Model file for the job. Use its own axes, mm. Face numbers are marked on the shaded views. A direction names the side the tool comes from. Round coordinates to 2 decimals unless told otherwise and drop trailing zeros. Order: outer loops, then holes, each group sorted by start corner. A loop starts at its lowest first (then second) coordinate and runs counter-clockwise, first axis right, second up. Notation, with made-up numbers: M -32.5,-37.75 L 10.5,-37.75 A8 ccw 10.5,-28.75 Z; hole C 39,74.25 d10. An arc over 180 degrees is marked long. Return JSON: item names as keys, results as strings. Group by question number.
Item 1: Slice it at D-D on y = 27.5. Write the cut outline in (x, z), then the cut area to 3 significant figures.
Item 2: Pull direction Z, two halves, no side cores. Call the marked faces 1, 2 and 3: pulls with the +Z half, pulls with the -Z half, needs draft (parallel to the pull), parting line crosses it, or undercut.
Item 3: Slice it at C-C on x = 7.5. Write the cut outline in (y, z).
Item 4: Slice it at A-A on x = -31.5. Write the cut outline in (y, z), then the cut area to 4 significant figures.
Item 5: Slice it at B-B on z = -40.5. Write the cut outline in (x, y), then the cut area to 3 significant figures.
Item 6: Probe line 1 along Z through (x, y) = (-55.5, 3.85); line 2 along X through (y, z) = (3.85, 69.5); line 3 along Y through (x, z) = (-22.5, 65.5). List the from-to ranges inside material, lowest first.
Item 7: Pin check, flat tips, straight feed: pin 1 Ø4.5 at (x, z) = (-55.5, 5.5) entering from -Y; pin 2 Ø13 at (y, z) = (38, 31.5) entering from -X; pin 3 Ø2 at (x, z) = (-38.5, 9.5) entering from +Y. Stop position of each tip, or through.
Item 8: Which spindle directions (+Z, -Z, +X, -X, +Y, -Y) get a long thin tool onto all of the face, cutting with end or side? Do the marked faces 4, 5 and 6. Say none if no direction does.
from build123d import *

# Parameters (mm, degrees)
SKETCH1_W                                           = 52
SKETCH1_H                                           = 100
BOSS_EXTRUDE1_DEPTH                                 = 5
BOSS_EXTRUDE3_DEPTH                                 = 2.5
SKETCH7_R                                           = 2.25
BOSS_EXTRUDE4_DEPTH                                 = 2.5
FILLET2_R                                           = 0.25
SKETCH9_W                                           = 52
SKETCH9_H                                           = 4
BOSS_EXTRUDE5_DEPTH                                 = 50
BOSS_EXTRUDE7_DEPTH                                 = 52
CUT_EXTRUDE3_DEPTH                                  = 52
CUT_EXTRUDE4_DEPTH                                  = 2.5
BOSS_EXTRUDE8_DEPTH                                 = 52
BOSS_EXTRUDE9_DEPTH                                 = 4
LPATTERN1_COUNT                                     = 2
LPATTERN1_PITCH                                     = 48
SKETCH18_R                                          = 11.5
CUT_EXTRUDE5_DEPTH                                  = 4
CSK_FOR_M3_COUNTERSUNK_FLAT_HEAD_SCREW1_D           = 3.4
CSK_FOR_M3_COUNTERSUNK_FLAT_HEAD_SCREW1_DEPTH       = 5
CSK_FOR_M3_COUNTERSUNK_FLAT_HEAD_SCREW1_CSINK_D     = 6.3
CSK_FOR_M3_COUNTERSUNK_FLAT_HEAD_SCREW1_CSINK_ANGLE = 90
CSK_FOR_M3_COUNTERSUNK_FLAT_HEAD_SCREW1_TIP         = 1.021463052
BOSS_EXTRUDE10_DEPTH                                = 5
SKETCH23_R                                          = 1.75
CUT_EXTRUDE6_DEPTH                                  = 5
SKETCH24_W                                          = 6.6
SKETCH24_H                                          = 5.6
CUT_EXTRUDE7_DEPTH                                  = 2.5


with BuildPart() as part:
    # Sketch1 → Boss-Extrude1 (new body)
    with BuildSketch(Plane(origin=(0, 0, 0), x_dir=(1, 0, 0), z_dir=(0, 1, 0))):
        Rectangle(SKETCH1_W, SKETCH1_H)
    extrude(amount=BOSS_EXTRUDE1_DEPTH)

    # Sketch2 → Boss-Extrude3 (add)
    with BuildSketch(Plane(origin=(0, 5, 0), x_dir=(1, 0, 0), z_dir=(0, 1, 0))):
        with BuildLine():
            Line((-26, 50), (26, 50))
            Line((26, 50), (26, 30))
            ThreePointArc((26, 30), (0, 22.708313008), (-26, 30))
            Line((-26, 30), (-26, 50))
        make_face()
    extrude(amount=BOSS_EXTRUDE3_DEPTH)

    # Sketch7 → Boss-Extrude4 (add)
    with BuildSketch(Plane(origin=(0, 7.5, 0), x_dir=(1, 0, 0), z_dir=(0, 1, 0))):
        with Locations((-7.5, 40.5)):
            Circle(SKETCH7_R)
        with Locations((7.5, 40.5)):
            Circle(SKETCH7_R)
    extrude(amount=BOSS_EXTRUDE4_DEPTH)

    # Fillet2
    fillet2_edges = [part.edges().sort_by_distance(p)[0] for p in [
        (-9.75, 10, -40.5),
        (5.25, 10, -40.5),
    ]]
    fillet(fillet2_edges, radius=FILLET2_R)

    # Sketch9 → Boss-Extrude5 (add)
    with BuildSketch(Plane(origin=(0, 5, 0), x_dir=(1, 0, 0), z_dir=(0, 1, 0))):
        with Locations((0, -2)):
            Rectangle(SKETCH9_W, SKETCH9_H)
    extrude(amount=BOSS_EXTRUDE5_DEPTH)

    # Sketch10 → Boss-Extrude7 (add)
    with BuildSketch(Plane.ZY.offset(26)):
        Polygon((4, 25), (25.126220325, 64.732641679), (21.594429954, 66.61052793), (4, 33.520217873), align=None)
    extrude(amount=-BOSS_EXTRUDE7_DEPTH)

    # Sketch11 → Cut-Extrude3 (cut)
    with BuildSketch(Plane.ZY.offset(26)):
        Polygon((4, 33.520217873), (0, 25.498656006), (0, 55), (4, 55), align=None)
    extrude(amount=-CUT_EXTRUDE3_DEPTH, mode=Mode.SUBTRACT)

    # Sketch13 → Cut-Extrude4 (cut)
    with BuildSketch(Plane(origin=(0, 7.5, 0), x_dir=(1, 0, 0), z_dir=(0, 1, 0))):
        with BuildLine():
            Line((-14.75, 24.933450371), (-14.75, 50))
            Line((-14.75, 50), (-26, 50))
            Line((-26, 50), (-26, 30))
            ThreePointArc((-26, 30), (-20.531880242, 27.118381074), (-14.75, 24.933450371))
        make_face()
        with BuildLine():
            Line((26, 50), (14.75, 50))
            Line((14.75, 50), (14.75, 24.933450371))
            ThreePointArc((14.75, 24.933450371), (20.531880242, 27.118381074), (26, 30))
            Line((26, 30), (26, 50))
        make_face()
    extrude(amount=-CUT_EXTRUDE4_DEPTH, mode=Mode.SUBTRACT)

    # Sketch16 → Boss-Extrude8 (add)
    with BuildSketch(Plane.ZY.offset(26)):
        Polygon((4.234735781, 25.441473796), (42.679556541, 5), (37.679556541, 5), (4, 22.907737867), (4, 25), align=None)
    extrude(amount=-BOSS_EXTRUDE8_DEPTH)

    # Sketch17 → Boss-Extrude9 (add)
    with BuildSketch(Plane.ZY.offset(26)):
        Polygon((25.126220325, 64.732641679), (25.126220325, 5), (20.126220325, 5), (20.126220325, 55.329009352), align=None)
    boss_extrude9 = extrude(amount=-BOSS_EXTRUDE9_DEPTH)

    # LPattern1: Boss-Extrude9 ×2
    with Locations(*[(i * LPATTERN1_PITCH, 0, 0) for i in range(1, LPATTERN1_COUNT)]):
        add(boss_extrude9)

    # Sketch18 → Cut-Extrude5 (cut)
    with BuildSketch(Plane(origin=(0, 5.729899813, -10.776374221), x_dir=(-1, 0, 0), z_dir=(0, 0.469471563, -0.882947593))):
        with Locations((0, 45.951576073)):
            Circle(SKETCH18_R)
    extrude(amount=-CUT_EXTRUDE5_DEPTH, mode=Mode.SUBTRACT)

    # CSK for M3 Countersunk Flat Head Screw1
    with Locations(Plane(origin=(0, 5.729899813, -10.776374221), x_dir=(-1, 0, 0), z_dir=(0, 0.469471563, -0.882947593))):
        with Locations((-15.5, 61.451576073), (15.5, 61.451576073), (15.5, 30.451576073), (-15.5, 30.451576073)):
            CounterSinkHole(CSK_FOR_M3_COUNTERSUNK_FLAT_HEAD_SCREW1_D / 2, CSK_FOR_M3_COUNTERSUNK_FLAT_HEAD_SCREW1_CSINK_D / 2, depth=CSK_FOR_M3_COUNTERSUNK_FLAT_HEAD_SCREW1_DEPTH, counter_sink_angle=CSK_FOR_M3_COUNTERSUNK_FLAT_HEAD_SCREW1_CSINK_ANGLE)
            with Locations((0, 0, -(CSK_FOR_M3_COUNTERSUNK_FLAT_HEAD_SCREW1_DEPTH + CSK_FOR_M3_COUNTERSUNK_FLAT_HEAD_SCREW1_TIP / 2))):  # 118° drill point
                Cone(0, CSK_FOR_M3_COUNTERSUNK_FLAT_HEAD_SCREW1_D / 2, CSK_FOR_M3_COUNTERSUNK_FLAT_HEAD_SCREW1_TIP, mode=Mode.SUBTRACT)

    # Sketch22 → Boss-Extrude10 (add)
    with BuildSketch(Plane.XZ):
        Polygon((26, 75), (-61, 75), (-61, 0), (-26, 0), (-26, 50), (26, 50), align=None)
    extrude(amount=-BOSS_EXTRUDE10_DEPTH)

    # Sketch23 → Cut-Extrude6 (cut)
    with BuildSketch(Plane(origin=(0, 5, 0), x_dir=(1, 0, 0), z_dir=(0, 1, 0))):
        with Locations((-31.5, -5.5)):
            Circle(SKETCH23_R)
        with Locations((-55.5, -5.5)):
            Circle(SKETCH23_R)
        with Locations((-55.5, -69.5)):
            Circle(SKETCH23_R)
        with Locations((-31.5, -69.5)):
            Circle(SKETCH23_R)
    extrude(amount=-CUT_EXTRUDE6_DEPTH, mode=Mode.SUBTRACT)

    # Sketch24 → Cut-Extrude7 (cut)
    with BuildSketch(Plane.XZ):
        with Locations((-31.5, 69.5)):
            Rectangle(SKETCH24_W, SKETCH24_H)
        with Locations((-55.5, 69.5)):
            Rectangle(SKETCH24_W, SKETCH24_H)
        with Locations((-31.5, 5.5)):
            Rectangle(SKETCH24_W, SKETCH24_H)
        with Locations((-55.5, 5.5)):
            Rectangle(SKETCH24_W, SKETCH24_H)
    extrude(amount=-CUT_EXTRUDE7_DEPTH, mode=Mode.SUBTRACT)


solid = part.part
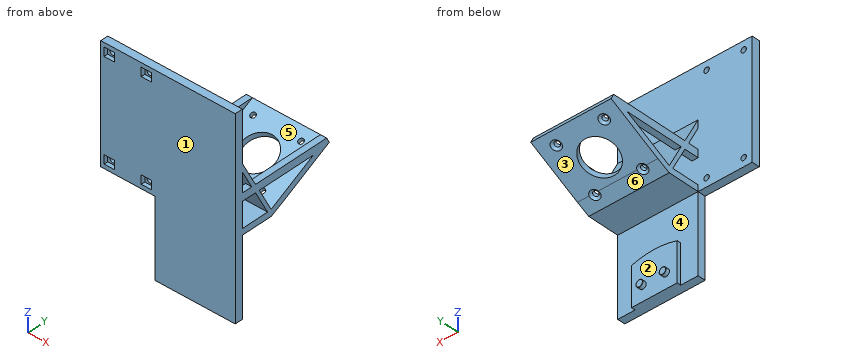
Output values:
{
 "1": {"outline": "M -26,1 L 26,1 L 26,5.33 L -26,5.33 Z; M -26,20.13 L -22,20.13 L -22,25.13 L -26,25.13 Z; M 22,20.13 L 26,20.13 L 26,25.13 L 22,25.13 Z", "area": "265 mm²"},
 "2": {"face 1": "needs draft", "face 2": "undercut", "face 3": "pulls with the -Z half"},
 "3": {"outline": "M 0,-50 L 7.5,-50 L 7.5,-42.75 L 9.75,-42.75 A0.25 ccw 10,-42.5 L 10,-38.5 A0.25 ccw 9.75,-38.25 L 7.5,-38.25 L 7.5,-23.27 L 5,-23.27 L 5,0 L 25.5,0 L 33.52,4 L 38.61,6.7 L 36.73,10.24 L 25.44,4.23 L 5,42.68 L 5,75 L 0,75 Z; M 52.12,18.42 L 54,14.89 L 66.61,21.59 L 64.73,25.13 Z; hole M 5,4 L 22.91,4 L 5,37.68 Z"},
 "4": {"outline": "M 0,0 L 5,0 L 5,3.75 L 2.5,3.75 L 2.5,2.7 L 0,2.7 Z; M 0,8.3 L 2.5,8.3 L 2.5,7.25 L 5,7.25 L 5,67.75 L 2.5,67.75 L 2.5,66.7 L 0,66.7 Z; M 0,72.3 L 2.5,72.3 L 2.5,71.25 L 5,71.25 L 5,75 L 0,75 Z", "area": "329.5 mm²"},
 "5": {"outline": "M -26,0 L 26,0 L 26,5 L 14.75,5 L 14.75,7.5 L 9.75,7.5 L 9.75,9.75 A0.25 ccw 9.5,10 L 5.5,10 A0.25 ccw 5.25,9.75 L 5.25,7.5 L -5.25,7.5 L -5.25,9.75 A0.25 ccw -5.5,10 L -9.5,10 A0.25 ccw -9.75,9.75 L -9.75,7.5 L -14.75,7.5 L -14.75,5 L -26,5 Z", "area": "356 mm²"},
 "6": {"line 1": "0 to 3.75, 7.25 to 67.75, 71.25 to 75", "line 2": "-61 to -57.25, -53.75 to -33.25, -29.75 to 26", "line 3": "0 to 5"},
 "7": {"pin 1": "y = 2.5", "pin 2": "x = -26", "pin 3": "y = 5"},
 "8": {"face 4": "+Y", "face 5": "none", "face 6": "-Z, +X, -X, +Y"}
}
